from build123d import *

# Parameters (mm, degrees)
CROQUIS1_R              = 6
CROQUIS1_R_2            = 4
SALIENTE_EXTRUIR1_DEPTH = 13
CROQUIS2_R              = 1.5
SALIENTE_EXTRUIR2_DEPTH = 5
CROQUIS3_R              = 1.5
CORTAR_EXTRUIR1_DEPTH   = 24


with BuildPart() as part:
    # Croquis1 → Saliente-Extruir1 (new body)
    with BuildSketch(Plane(origin=(0, 0, 0), x_dir=(1, 0, 0), z_dir=(0, 1, 0))):
        with Locations(Location((0, 0, 0), (0, 0, 90))):
            Circle(CROQUIS1_R)
        with Locations(Location((0, 0, 0), (0, 0, 90))):
            Circle(CROQUIS1_R_2, mode=Mode.SUBTRACT)
    extrude(amount=SALIENTE_EXTRUIR1_DEPTH)

    # Croquis2 → Saliente-Extruir2 (add)
    with BuildSketch(Plane(origin=(0, 13, 0), x_dir=(1, 0, 0), z_dir=(0, 1, 0))):
        Polygon((6.17109675, -3.149216553), (5.812849912, 3.769718279), (-0.358246838, 6.918934832), (-6.17109675, 3.149216553), (-5.812849912, -3.769718279), (0.358246838, -6.918934832), align=None)
        with Locations(Location((0, 0, 0), (0, 0, 270))):
            Circle(CROQUIS2_R, mode=Mode.SUBTRACT)
    extrude(amount=SALIENTE_EXTRUIR2_DEPTH)

    # Croquis3 → Cortar-Extruir1 (cut)
    with BuildSketch(Plane(origin=(-5.991973331, 0, 0.310250863), x_dir=(0.0517084771330075, 0, 0.9986622218711316), z_dir=(-0.9986622218711316, 0, 0.0517084771330075))):
        with Locations((-0.007268939, 6.5)):
            Circle(CROQUIS3_R)
    extrude(amount=-CORTAR_EXTRUIR1_DEPTH, mode=Mode.SUBTRACT)


solid = part.part
Verification items for the finished model (mm, model axes). A direction names the side the tool comes from. Coordinates: 2 decimals unless noted, no trailing zeros. Order: outer loops, then holes, each group sorted by start corner. A loop starts at its lowest first (then second) coordinate and runs counter-clockwise, first axis right, second up. Notation, with made-up numbers: M 32.5,24.25 L 91.5,24.25 A23 ccw 91.5,58.25 Z; hole C 45.5,-23 d10. An arc over 180 degrees is marked long. Return JSON: item names as keys, results as strings.
1) Release check for a two-part mould opening along Z. For faces 1 (the cylindrical face through (3.549, 6.409, -1.846)), 2 (the flat face through (0, 18, -2)), 3 (the flat face through (2.77, 15.465, -5.322)) record: +Z half, -Z half, draft (parallel to the pull), parting line (faces both ways), or undercut.
Answer list:
{"face 1": "undercut", "face 2": "draft", "face 3": "-Z half"}
2) Gauge pin test, flat ends, axial feed: pin 1 (5 mm diameter, centred on x = 0, z = 0, fed in from -Y); pin 2 (0.6 mm diameter, centred on x = -0.5, z = 5.5, fed in from -Y); pin 3 (5 mm diameter, centred on y = 3, z = -3, fed in from -X); pin 4 (1.5 mm diameter, centred on x = 4, y = 14, fed in from +Z). Record the tip position at first contact, or that the pin passes through.
Answer list:
{"pin 1": "y = 13", "pin 2": "y = 0", "pin 3": "x = -5.98", "pin 4": "z = 5.04"}
3) Cross-section at A-A, the plane y = 15. Record the boundary of the cut face in (x, z).
Answer list:
{"outline": "M -6.17,-3.15 L -0.36,-6.92 L 5.81,-3.77 L 6.17,3.15 L 0.36,6.92 L -5.81,3.77 Z; hole C 0,0 d3"}
4) Access from +Z, -Z, +X, -X, +Y, -Y to the whole of each face (thin tool, end or side, straight path). Record for faces 4 (the flat face through (2, 13, 0)), 5 (the flat face through (-6, 13, -3)), 6 (the flat face through (-5.2, 13, 3.4)), 7 (the flat face through (5.2, 13, -3.4)).
Answer list:
{"face 4": "-Y", "face 5": "-Z, -X, -Y", "face 6": "+Z, -X, -Y", "face 7": "-Z, +X, -Y"}
5) Cross-section at C-C, the plane z = -3.5. Record the boundary of the cut face in (x, y), and give its area (3 significant figures).
Answer list:
{"outline": "M -5.63,13 L -4.87,13 L -4.87,0 L -1.94,0 L -1.94,13 L 1.94,13 L 1.94,0 L 4.87,0 L 4.87,13 L 5.83,13 L 5.83,18 L -5.63,18 Z", "area": "134 mm2"}
6) Thickness scan on L1, parallel to X at y = 3.25, z = 0; L2, parallel to X at y = 14.35, z = 0; L3, parallel to Z at x = 3, y = 5.5. Record the ranges inside material, lowest first. Write a range as [from, to].
Answer list:
{"L1": "[-6, -4], [4, 6]", "L2": "[-6.01, -1.5], [1.5, 6.01]", "L3": "[-5.2, -2.65], [2.65, 5.2]"}
7) Cross-section at B-B, the plane x = 0. Record the boundary of the cut face in (y, z), and give its area (3 significant figures).
Answer list:
{"outline": "M 0,-6 L 13,-6 L 13,-6.74 L 18,-6.74 L 18,-1.5 L 13,-1.5 L 13,-4 L 0,-4 Z; M 0,4 L 13,4 L 13,1.5 L 18,1.5 L 18,6.74 L 13,6.74 L 13,6 L 0,6 Z", "area": "104 mm2"}
